Verification items for the finished model (mm, model axes). A direction names the side the tool comes from. Give positions to 0.01 mm unless a question says otherwise; leave off trailing zeros. Order: outer loops, then holes, each group sorted by start corner. A loop starts at its lowest first (then second) coordinate and runs counter-clockwise, first axis right, second up.
from build123d import *

# Parameters (mm, degrees)
BOSS_EXTRUDE1_DEPTH     = 300
SKETCH3_W               = 200
SKETCH3_H               = 20
BOSS_EXTRUDE3_DEPTH     = 90
CUT_EXTRUDE1_DEPTH      = 311.64449134
CUT_EXTRUDE1_DEPTH_BACK = 311.64449134
SKETCH5_W               = 200.997512422
SKETCH5_H               = 300
BOSS_EXTRUDE4_DEPTH     = 13.35
BOSS_EXTRUDE5_DEPTH     = 300
CUT_EXTRUDE2_START      = 100
CUT_EXTRUDE2_OUTLINE_W  = 16
CUT_EXTRUDE2_OUTLINE_H  = 302
CUT_EXTRUDE2_DEPTH      = 2
BOSS_EXTRUDE6_DEPTH     = 20
SKETCH9_W               = 20
SKETCH9_H               = 150
BOSS_EXTRUDE7_DEPTH     = 100
SKETCH10_W              = 20
SKETCH10_H              = 120.070032415
BOSS_EXTRUDE8_DEPTH     = 5


with BuildPart() as part:
    # Sketch2 → Boss-Extrude1 (new body)
    with BuildSketch(Plane.XY):
        Polygon((-100, -10), (-100, -16.653448461), (100, 3.346551539), (100, 10), align=None)
    extrude(amount=BOSS_EXTRUDE1_DEPTH)

    # Sketch3 → Boss-Extrude3 (add, symmetric)
    with BuildSketch(Plane(origin=(0, 0, 0), x_dir=(1, 0, 0), z_dir=(0, 1, 0))):
        with Locations((0, -10)):
            Rectangle(SKETCH3_W, SKETCH3_H)
        with Locations((0, -290)):
            Rectangle(SKETCH3_W, SKETCH3_H)
    extrude(amount=BOSS_EXTRUDE3_DEPTH, both=True)

    # Sketch4 → Cut-Extrude1 (cut, two sides: drawn at the far end of the back side and taken through both)
    with BuildSketch(Plane.XY.offset(20).offset(-CUT_EXTRUDE1_DEPTH_BACK)):
        Polygon((-100, -16.653448461), (-100, -90), (100, -90), (100, 3.346551539), align=None)
    extrude(amount=CUT_EXTRUDE1_DEPTH + CUT_EXTRUDE1_DEPTH_BACK, mode=Mode.SUBTRACT)

    # Sketch5 → Boss-Extrude4 (add)
    with BuildSketch(Plane(origin=(0.658757273, -6.587572734, 0), x_dir=(0.9950371902099892, 0.09950371902099911, 0), z_dir=(0.09950371902099912, -0.9950371902099893, 0))):
        with Locations((-0.662042866, 150)):
            Rectangle(SKETCH5_W, SKETCH5_H)
    extrude(amount=BOSS_EXTRUDE4_DEPTH)

    # Boss-Extrude5: read off the stored shape, not the designer's step
    # Boss-Extrude5 outline → Boss-Extrude5 (add)
    with BuildSketch(Plane.XY):
        Polygon((-100, -16.653448461), (-100, -30.070032415), (-98.671625351, -29.93719495), align=None)
    extrude(amount=BOSS_EXTRUDE5_DEPTH)

    # Cut-Extrude2: read off the stored shape, not the designer's step
    # Cut-Extrude2 outline → Cut-Extrude2 (cut)
    with BuildSketch(Plane.YZ.offset(CUT_EXTRUDE2_START)):
        with Locations((-3, 150)):
            Rectangle(CUT_EXTRUDE2_OUTLINE_W, CUT_EXTRUDE2_OUTLINE_H)
    extrude(amount=CUT_EXTRUDE2_DEPTH, mode=Mode.SUBTRACT)

    # Sketch8 → Boss-Extrude6 (add)
    with BuildSketch(Plane.ZY.offset(100)):
        Polygon((300, 90), (280, 90), (280, -10), (130, -10), (130, -30.070032415), (300, -30.070032415), align=None)
    extrude(amount=BOSS_EXTRUDE6_DEPTH)

    # Sketch9 → Boss-Extrude7 (add)
    with BuildSketch(Plane(origin=(0, -10, 0), x_dir=(1, 0, 0), z_dir=(0, 1, 0))):
        with Locations((-110, -205)):
            Rectangle(SKETCH9_W, SKETCH9_H)
    extrude(amount=BOSS_EXTRUDE7_DEPTH)

    # Sketch10 → Boss-Extrude8 (add)
    with BuildSketch(Plane(origin=(0, 0, 130), x_dir=(-1, 0, 0), z_dir=(0, 0, -1))):
        with Locations((110, 29.964983792)):
            Rectangle(SKETCH10_W, SKETCH10_H)
    extrude(amount=BOSS_EXTRUDE8_DEPTH)


solid = part.part
(1) Section check B-B, the plane y = 6. Enter the section's corners in (x, z).
Solved:
outline: (-120, 125) - (-100, 125) - (-100, 280) - (60, 280) - (60, 20) - (-100, 20) - (-100, 0) - (100, 0) - (100, 300) - (-120, 300) - close
(2) Section check D-D, the plane x = 81. Enter the section's corners in (y, z).
Solved:
outline: (-11.97, 0) - (90, 0) - (90, 20) - (8.1, 20) - (8.1, 280) - (90, 280) - (90, 300) - (-11.97, 300) - close
(3) Section check A-A, the plane y = 53. Enter the section's corners in (x, z), then the cut area to 3 significant figures.
Solved:
outline: (-120, 125) - (-100, 125) - (-100, 280) - (100, 280) - (100, 300) - (-120, 300) - close; (-100, 0) - (100, 0) - (100, 20) - (-100, 20) - close
area: 11,500 mm2
(4) Section check C-C, the plane z = 141. Enter the section's corners in (x, y), then the cut area to 3 significant figures.
Solved:
outline: (-120, -30.07) - (-100, -30.07) - (100, -10.07) - (100, 10) - (-100, -10) - (-100, 90) - (-120, 90) - close
area: 6,420 mm2
(5) Release check for a two-part mould opening along Z. For faces 1 (the flat face through (-100, 4, 16)), 2 (the flat face through (-110, 31, 125)), 3 (the flat face through (1, 41, 280)) record: pulls with the +Z half, pulls with the -Z half, needs draft (parallel to the pull), parting line crosses it, or undercut.
Solved:
face 1: needs draft
face 2: pulls with the -Z half
face 3: undercut
(6) Go/stop test with flat-tipped pins: pin 1 (4 mm diameter, centred on x = -32.5, z = 148.5, fed in from +Y); pin 2 (3 mm diameter, centred on x = 4.5, z = 32.5, fed in from -Y); pin 3 (4 mm diameter, centred on x = -92.5, z = 261.5, fed in from +Y). Record where each tip stops, or that it passes through.
Solved:
pin 1: stops at y = -3.05
pin 2: stops at y = -19.77
pin 3: stops at y = -9.05
(7) Scan lines: line 1 (Z direction, x = 42.5, y = 41.5); line 2 (Z direction, x = -103.5, y = 29); line 3 (X direction, y = 42, z = 230). Record each from-to range of solid material in increasing order.
Solved:
line 1: z = 0 to 20, 280 to 300
line 2: z = 125 to 300
line 3: x = -120 to -100
(8) Set-up check for faces 4 (the flat face through (-100, 39, 204)), 5 (the flat face through (100, 7, 152)), 6 (the flat face through (-1, 39, 20)): record each of +Z, -Z, +X, -X, +Y, -Y from which the full face is reachable in a straight line by a thin tool's end or side.
Solved:
face 4: +Y
face 5: +Z, -Z, +X, +Y, -Y
face 6: -X, +Y
